```python
from build123d import *

# Parameters (mm, degrees)
SKETCH_1_R          = 52
SKETCH_1_R_2        = 29
SKETCH_1_R_3        = 2.05
EXTRUDE_1_DEPTH     = 2.5
SKETCH_2_W          = 182
SKETCH_2_H          = 210.035227354
SKETCH_2_W_2        = 82
SKETCH_2_H_2        = 110.035227354
CUT_EXTRUDE_1_DEPTH = 4


with BuildPart() as part:
    # 草图1 → 凸台-拉伸1 (new body)
    with BuildSketch(Plane(origin=(0, 0, 0), x_dir=(1, 0, 0), z_dir=(0, 1, 0))):
        with Locations(Location((0, 0, 0), (0, 0, 270))):
            Circle(SKETCH_1_R)
        with Locations(Location((0, 0, 0), (0, 0, 270))):
            Circle(SKETCH_1_R_2, mode=Mode.SUBTRACT)
        with Locations(Location((47, 0, 0), (0, 0, 270))):
            Circle(SKETCH_1_R_3, mode=Mode.SUBTRACT)
        with Locations(Location((33.234018716, -33.234018716, 0), (0, 0, 270))):
            Circle(SKETCH_1_R_3, mode=Mode.SUBTRACT)
        with Locations(Location((0, -47, 0), (0, 0, 270))):
            Circle(SKETCH_1_R_3, mode=Mode.SUBTRACT)
        with Locations(Location((-33.234018716, -33.234018716, 0), (0, 0, 270))):
            Circle(SKETCH_1_R_3, mode=Mode.SUBTRACT)
        with Locations(Location((-47, 0, 0), (0, 0, 270))):
            Circle(SKETCH_1_R_3, mode=Mode.SUBTRACT)
        with Locations(Location((-33.234018716, 33.234018716, 0), (0, 0, 270))):
            Circle(SKETCH_1_R_3, mode=Mode.SUBTRACT)
        with Locations(Location((0, 47, 0), (0, 0, 270))):
            Circle(SKETCH_1_R_3, mode=Mode.SUBTRACT)
        with Locations(Location((33.234018716, 33.234018716, 0), (0, 0, 270))):
            Circle(SKETCH_1_R_3, mode=Mode.SUBTRACT)
    extrude(amount=EXTRUDE_1_DEPTH)

    # 草图2 → 切除-拉伸-薄壁1 (cut)
    with BuildSketch(Plane(origin=(0, 2.5, 0), x_dir=(1, 0, 0), z_dir=(0, 1, 0))):
        Rectangle(SKETCH_2_W, SKETCH_2_H)
        Rectangle(SKETCH_2_W_2, SKETCH_2_H_2, mode=Mode.SUBTRACT)
    extrude(amount=-CUT_EXTRUDE_1_DEPTH, mode=Mode.SUBTRACT)


solid = part.part
```
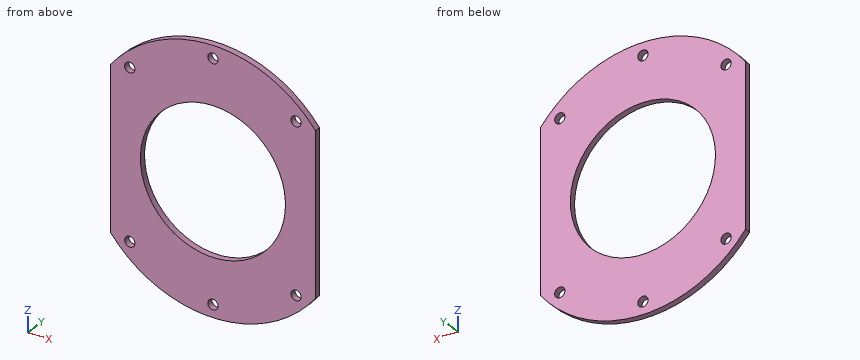
The listing builds one solid part. Answer for the finished solid, in the listing's coordinates (mm). Give positions to 0.01 mm unless a question says otherwise; leave off trailing zeros. Order: outer loops, then holes, each group sorted by start corner. A loop starts at its lowest first (then second) coordinate and runs counter-clockwise, first axis right, second up. Notation, with made-up numbers: M -33,36 L -15,36 A29 cw -15,61 Z; hole C 66,-27.5 d11. An arc over 180 degrees is marked long. Put each result on its own line as item: value. Start each with the question number.
Item 1: The part is cut by section C-C, the plane x = 17. Determine the outline of the cut face in (y, z), and give its area (3 significant figures).
Item 2: Find the intervals of material crossed by line 1 along X through (y, z) = (1.7, -19.5); line 2 along X through (y, z) = (0.7, -22.5); line 3 along Z through (x, y) = (20, 2.1), in increasing order.
Item 3: The part is cut by section B-B, the plane x = 0. Determine the outline of the cut face in (y, z), and give its area (3 significant figures).
Item 4: The part is cut by section A-A, the plane z = 0. Determine the outline of the cut face in (x, y).
Item 5: The part is cut by section D-D, the plane z = -34. Determine the outline of the cut face in (x, y), and give its area (3 significant figures).
Item 6: Flat-ended cylindrical pins translate along their axes: P1, Ø3, axis at x = 20.5, z = -31.5, coming from the -Y side; P2, Ø1, axis at x = 10, y = 2, coming from the +Z side; P3, Ø2.5, axis at x = -33.23, z = 33.23, coming from the -Y side. Find the tip coordinate at first contact, or state that the pin passes through.
Answer key:
1. outline: M 0,-49.14 L 2.5,-49.14 L 2.5,-23.49 L 0,-23.49 Z; M 0,23.49 L 2.5,23.49 L 2.5,49.14 L 0,49.14 Z
1. area: 128 mm²
2. line 1: x = -41 to -21.47, 21.47 to 41
2. line 2: x = -41 to -18.3, 18.3 to 41
2. line 3: z = -48 to -21, 21 to 48
3. outline: M 0,-52 L 2.5,-52 L 2.5,-49.05 L 0,-49.05 Z; M 0,-44.95 L 2.5,-44.95 L 2.5,-29 L 0,-29 Z; M 0,29 L 2.5,29 L 2.5,44.95 L 0,44.95 Z; M 0,49.05 L 2.5,49.05 L 2.5,52 L 0,52 Z
3. area: 94.5 mm²
4. outline: M -41,0 L -29,0 L -29,2.5 L -41,2.5 Z; M 29,0 L 41,0 L 41,2.5 L 29,2.5 Z
5. outline: M -39.34,0 L -35.14,0 L -35.14,2.5 L -39.34,2.5 Z; M -31.33,0 L 31.33,0 L 31.33,2.5 L -31.33,2.5 Z; M 35.14,0 L 39.34,0 L 39.34,2.5 L 35.14,2.5 Z
5. area: 178 mm²
6. P1: stops at y = 0
6. P2: stops at z = 51.12
6. P3: passes through
